Autodesk Inventor part; units mm, degrees
ref_plane "Work Plane1" through (-28.4804, 33.3109, -32.5631) normal (-1, 0, 0) x (0, 0, 1)
ref_plane "YZ Plane" through (0, 0, 0) normal (1, 0, 0) x (0, 1, 0)
ref_plane "XZ Plane" through (0, 0, 0) normal (0, 1, 0) x (-1, 0, 0)
sketch "Sketch1" plane through (0, 0, 0) normal (0, 0, 1) x (1, 0, 0)
  line L0 (6.9956, 3.6314) -> (6.4167, 3.8711)
  line L1 (5.7956, 3.9529) -> (6.4167, 3.8711)
  line L2 (5.1744, 3.8711) -> (5.7956, 3.9529)
  line L3 (4.5956, 3.6314) -> (5.1744, 3.8711)
  line L4 (4.0985, 3.25) -> (4.5956, 3.6314)
  line L5 (3.7171, 2.7529) -> (4.0985, 3.25)
  line L6 (3.4773, 2.1741) -> (3.7171, 2.7529)
  line L7 (3.4773, 2.1741) -> (3.3956, 1.5529)
  line L8 (3.4773, 0.9317) -> (3.3956, 1.5529)
  line L9 (3.4773, 0.9317) -> (3.7171, 0.3529)
  line L10 (3.7171, 0.3529) -> (4.0985, -0.1441)
  line L11 (4.0985, -0.1441) -> (4.5956, -0.5255)
  line L12 (4.5956, -0.5255) -> (5.1744, -0.7653)
  line L13 (5.1744, -0.7653) -> (5.7956, -0.8471)
  line L14 (5.7956, -0.8471) -> (6.4167, -0.7653)
  line L15 (6.4167, -0.7653) -> (6.9956, -0.5255)
  line L16 (6.9956, -0.5255) -> (7.4926, -0.1441)
  line L17 (7.4926, -0.1441) -> (7.874, 0.3529)
  line L18 (8.1138, 0.9317) -> (7.874, 0.3529)
  line L19 (8.1138, 0.9317) -> (8.1956, 1.5529)
  line L20 (8.1956, 1.5529) -> (8.1138, 2.1741)
  line L21 (8.1138, 2.1741) -> (7.874, 2.7529)
  line L22 (7.874, 2.7529) -> (7.4926, 3.25)
  line L23 (6.9956, 3.6314) -> (7.4926, 3.25)
  line L24 (6.7956, 1.5529) -> (6.7615, 1.8117)
  line L25 (6.7615, 1.2941) -> (6.7956, 1.5529)
  line L26 (6.6616, 1.0529) -> (6.7615, 1.2941)
  line L27 (6.5027, 0.8458) -> (6.6616, 1.0529)
  line L28 (6.2956, 0.6869) -> (6.5027, 0.8458)
  line L29 (6.0544, 0.587) -> (6.2956, 0.6869)
  line L30 (5.7956, 0.5529) -> (6.0544, 0.587)
  line L31 (5.5367, 0.587) -> (5.7956, 0.5529)
  line L32 (5.2956, 0.6869) -> (5.5367, 0.587)
  line L33 (5.0884, 0.8458) -> (5.2956, 0.6869)
  line L34 (4.9295, 1.0529) -> (5.0884, 0.8458)
  line L35 (4.8296, 1.2941) -> (4.9295, 1.0529)
  line L36 (4.7956, 1.5529) -> (4.8296, 1.2941)
  line L37 (4.7956, 1.5529) -> (4.8296, 1.8117)
  line L38 (4.8296, 1.8117) -> (4.9295, 2.0529)
  line L39 (4.9295, 2.0529) -> (5.0884, 2.26)
  line L40 (5.0884, 2.26) -> (5.2956, 2.4189)
  line L41 (5.2956, 2.4189) -> (5.5367, 2.5188)
  line L42 (5.5367, 2.5188) -> (5.7956, 2.5529)
  line L43 (5.7956, 2.5529) -> (6.0544, 2.5188)
  line L44 (6.0544, 2.5188) -> (6.2956, 2.4189)
  line L45 (6.2956, 2.4189) -> (6.5027, 2.26)
  line L46 (6.5027, 2.26) -> (6.6616, 2.0529)
  line L47 (6.6616, 2.0529) -> (6.7615, 1.8117)
  circle A0 centre (5.7956, 1.5529) radius 2.5
  arc A1 (1.7956, 7.8972) -> (9.7955, 7.8972) centre (5.7956, 1.5529) ccw
  line L48 (-28.4804, 55.5109) -> (-15.9804, 55.5109)
  line L49 (-28.4804, 55.5109) -> (-28.4804, 40.3109)
  line L50 (-15.9804, 40.3109) -> (-28.4804, 40.3109)
  line L51 (-15.9804, 40.3109) -> (-15.9804, 55.5109)
  line L52 (-20.6474, 51.7815) -> (-20.6304, 51.9109)
  line L53 (-20.6974, 51.6609) -> (-20.6474, 51.7815)
  line L54 (-20.7768, 51.5573) -> (-20.6974, 51.6609)
  line L55 (-20.8804, 51.4779) -> (-20.7768, 51.5573)
  line L56 (-21.001, 51.4279) -> (-20.8804, 51.4779)
  line L57 (-21.1304, 51.4109) -> (-21.001, 51.4279)
  line L58 (-21.2598, 51.4279) -> (-21.1304, 51.4109)
  line L59 (-21.3804, 51.4779) -> (-21.2598, 51.4279)
  line L60 (-21.4839, 51.5573) -> (-21.3804, 51.4779)
  line L61 (-21.5634, 51.6609) -> (-21.4839, 51.5573)
  line L62 (-21.5634, 51.6609) -> (-21.6133, 51.7815)
  line L63 (-21.6133, 51.7815) -> (-21.6304, 51.9109)
  line L64 (-21.6304, 51.9109) -> (-21.6133, 52.0403)
  line L65 (-21.5634, 52.1609) -> (-21.6133, 52.0403)
  line L66 (-21.4839, 52.2645) -> (-21.5634, 52.1609)
  line L67 (-21.3804, 52.3439) -> (-21.4839, 52.2645)
  line L68 (-21.3804, 52.3439) -> (-21.2598, 52.3939)
  line L69 (-21.2598, 52.3939) -> (-21.1304, 52.4109)
  line L70 (-21.1304, 52.4109) -> (-21.001, 52.3939)
  line L71 (-21.001, 52.3939) -> (-20.8804, 52.3439)
  line L72 (-20.8804, 52.3439) -> (-20.7768, 52.2645)
  line L73 (-20.7768, 52.2645) -> (-20.6974, 52.1609)
  line L74 (-20.6974, 52.1609) -> (-20.6474, 52.0403)
  line L75 (-20.6304, 51.9109) -> (-20.6474, 52.0403)
  line L76 (-21.7474, 51.7815) -> (-21.7304, 51.9109)
  line L77 (-21.7974, 51.6609) -> (-21.7474, 51.7815)
  line L78 (-21.8768, 51.5573) -> (-21.7974, 51.6609)
  line L79 (-21.9804, 51.4779) -> (-21.8768, 51.5573)
  line L80 (-22.101, 51.4279) -> (-21.9804, 51.4779)
  line L81 (-22.2304, 51.4109) -> (-22.101, 51.4279)
  line L82 (-22.3598, 51.4279) -> (-22.2304, 51.4109)
  line L83 (-22.4804, 51.4779) -> (-22.3598, 51.4279)
  line L84 (-22.5839, 51.5573) -> (-22.4804, 51.4779)
  line L85 (-22.6634, 51.6609) -> (-22.5839, 51.5573)
  line L86 (-22.6634, 51.6609) -> (-22.7133, 51.7815)
  line L87 (-22.7133, 51.7815) -> (-22.7304, 51.9109)
  line L88 (-22.7304, 51.9109) -> (-22.7133, 52.0403)
  line L89 (-22.6634, 52.1609) -> (-22.7133, 52.0403)
  line L90 (-22.5839, 52.2645) -> (-22.6634, 52.1609)
  line L91 (-22.4804, 52.3439) -> (-22.5839, 52.2645)
  line L92 (-22.4804, 52.3439) -> (-22.3598, 52.3939)
  line L93 (-22.3598, 52.3939) -> (-22.2304, 52.4109)
  line L94 (-22.2304, 52.4109) -> (-22.101, 52.3939)
  line L95 (-22.101, 52.3939) -> (-21.9804, 52.3439)
  line L96 (-21.9804, 52.3439) -> (-21.8768, 52.2645)
  line L97 (-21.8768, 52.2645) -> (-21.7974, 52.1609)
  line L98 (-21.7974, 52.1609) -> (-21.7474, 52.0403)
  line L99 (-21.7304, 51.9109) -> (-21.7474, 52.0403)
  line L100 (-22.8474, 51.7815) -> (-22.8304, 51.9109)
  line L101 (-22.8974, 51.6609) -> (-22.8474, 51.7815)
  line L102 (-22.9768, 51.5573) -> (-22.8974, 51.6609)
  line L103 (-23.0804, 51.4779) -> (-22.9768, 51.5573)
  line L104 (-23.201, 51.4279) -> (-23.0804, 51.4779)
  line L105 (-23.3304, 51.4109) -> (-23.201, 51.4279)
  line L106 (-23.4598, 51.4279) -> (-23.3304, 51.4109)
  line L107 (-23.5804, 51.4779) -> (-23.4598, 51.4279)
  line L108 (-23.6839, 51.5573) -> (-23.5804, 51.4779)
  line L109 (-23.7634, 51.6609) -> (-23.6839, 51.5573)
  line L110 (-23.7634, 51.6609) -> (-23.8133, 51.7815)
  line L111 (-23.8133, 51.7815) -> (-23.8304, 51.9109)
  line L112 (-23.8304, 51.9109) -> (-23.8133, 52.0403)
  line L113 (-23.7634, 52.1609) -> (-23.8133, 52.0403)
  line L114 (-23.6839, 52.2645) -> (-23.7634, 52.1609)
  line L115 (-23.5804, 52.3439) -> (-23.6839, 52.2645)
  line L116 (-23.5804, 52.3439) -> (-23.4598, 52.3939)
  line L117 (-23.4598, 52.3939) -> (-23.3304, 52.4109)
  line L118 (-23.3304, 52.4109) -> (-23.201, 52.3939)
  line L119 (-23.201, 52.3939) -> (-23.0804, 52.3439)
  line L120 (-23.0804, 52.3439) -> (-22.9768, 52.2645)
  line L121 (-22.9768, 52.2645) -> (-22.8974, 52.1609)
  line L122 (-22.8974, 52.1609) -> (-22.8474, 52.0403)
  line L123 (-22.8304, 51.9109) -> (-22.8474, 52.0403)
  line L124 (-21.6304, 37.8109) -> (-21.6304, 40.3109)
  line L125 (-15.9804, 37.8109) -> (-21.6304, 37.8109)
  line L126 (-15.9804, 37.8109) -> (-15.9804, 40.3109)
  line L127 (-21.6304, 40.3109) -> (-15.9804, 40.3109)
  line L128 (-28.4804, 37.8109) -> (-28.4804, 40.3109)
  line L129 (-22.8304, 37.8109) -> (-28.4804, 37.8109)
  line L130 (-22.8304, 37.8109) -> (-22.8304, 40.3109)
  line L131 (-28.4804, 40.3109) -> (-22.8304, 40.3109)
  line L132 (-28.4804, 40.3109) -> (-15.9804, 40.3109)
  line L133 (-15.9804, 40.3109) -> (-15.9804, 45.3109)
  line L134 (-15.9804, 45.3109) -> (-28.4804, 45.3109)
  line L135 (-28.4804, 45.3109) -> (-28.4804, 40.3109)
  line L136 (-15.9804, 45.3109) -> (-12.9804, 45.3109)
  line L137 (-12.9804, 45.3109) -> (-12.9804, 40.3109)
  line L138 (-12.9804, 40.3109) -> (-15.9804, 40.3109)
  line L139 (-15.9804, 40.3109) -> (-15.9804, 45.3109)
  line L140 (-28.4804, 45.3109) -> (-31.4804, 45.3109)
  line L141 (-31.4804, 45.3109) -> (-31.4804, 40.3109)
  line L142 (-31.4804, 40.3109) -> (-28.4804, 40.3109)
  line L143 (-28.4804, 40.3109) -> (-28.4804, 45.3109)
  line L144 (-12.9804, 45.3109) -> (5.7956, 45.3109)
  line L145 (1.7956, 40.3109) -> (-12.9804, 40.3109)
  line L146 (-12.9804, 40.3109) -> (-12.9804, 45.3109)
  line L147 (9.7956, 45.3109) -> (9.7955, 7.8972)
  line L148 (1.7956, 7.8972) -> (1.7956, 40.3109)
  line L149 (1.7956, 45.3109) -> (9.7956, 45.3109)
  line L150 (9.7956, 45.3109) -> (1.7956, 3.9529) construction
  line L151 (9.7956, 3.9529) -> (1.7956, 45.3109) construction
  line L152 (5.7956, 4.0529) -> (5.7956, 3.9529)
  line L153 (5.7956, 1.5529) -> (-36.8703, 1.5529)
  line L154 (-22.2304, 45.3109) -> (-22.2304, 1.5529)
  line L155 (1.7956, 39.0609) -> (1.7956, 45.3109)
  point P0 (0, 0)
  point P1 (5.7956, 24.6319)
  dimension "d0" = 5
  dimension "d1" = 15
  dimension "d2" = 5
  dimension "d3" = 3
  dimension "d4" = 3
  dimension "d6" = 8
extrude "Extrusion1" add sketch "Sketch1" along normal blind 3 contours A1 L148 L155 L144 L149 L147
sketch "Sketch2" plane through (1.7956, 39.0609, 0) normal (-1, 0, 0) x (0, 0, 1)
  line L0 (-5.2631, 16.45) -> (-5.2631, 1.25)
  line L1 (-27.7631, 1.25) -> (-27.7631, 16.45)
  line L2 (-5.2631, 16.45) -> (-27.7631, 16.45)
  line L3 (-27.7631, 1.25) -> (-27.7631, 16.45)
  line L4 (-27.7631, 1.25) -> (-32.5631, 1.25)
  line L5 (-32.5631, 1.25) -> (-32.5631, -1.25)
  line L6 (-27.7631, -1.25) -> (-32.5631, -1.25)
  line L7 (-27.7631, -1.25) -> (-27.7631, -5.75)
  line L8 (-5.2631, -5.75) -> (-27.7631, -5.75)
  line L9 (-5.2631, -1.25) -> (-5.2631, -5.75)
  line L10 (-5.2631, -1.25) -> (-0.4631, -1.25)
  line L11 (-0.4631, -1.25) -> (-0.4631, 1.25)
  line L12 (-5.2631, 1.25) -> (-0.4631, 1.25)
  line L13 (-5.2631, 16.45) -> (-5.2631, 1.25)
  line L14 (0, 6.25) -> (0, 0)
  line L15 (-27.7631, 1.25) -> (0, 1.25)
  line L16 (0, 1.25) -> (0, 6.25)
  line L17 (0, 6.25) -> (-27.7631, 6.25)
  line L18 (-27.7631, 6.25) -> (-27.7631, 1.25)
  line L19 (-27.7631, 6.25) -> (-30.7631, 6.25)
  line L20 (-30.7631, 6.25) -> (-30.7631, 1.25)
  line L21 (-30.7631, 1.25) -> (-27.7631, 1.25)
  line L22 (-27.7631, 1.25) -> (-27.7631, 6.25)
  point P0 (0, -39.0609)
  dimension "d9" = 3
ref_plane "Work Plane1" through (-28.4804, 33.3109, -32.5631) normal (-1, 0, 0) x (0, 0, 1)
extrude "Extrusion2" add sketch "Sketch2" against normal blind 15.5 from surface at 30.276 contours L17 L14 L15 L12 L0 | L0 L15 L1 L17
sketch "Sketch3" plane through (-12.9804, 40.3109, 0) normal (1, 0, 0) x (0, 0, -1)
  line L0 (0, -32.4137) -> (0, 5)
  line L1 (0, 5) -> (-3, 5)
  line L2 (-3, -32.4137) -> (-3, 5)
  line L3 (0, -32.4137) -> (-3, -32.4137)
  line L4 (0, 5) -> (0, 0)
  line L5 (0, 0) -> (27.7631, 0)
  line L6 (27.7631, 0) -> (27.7631, 5)
  line L7 (27.7631, 5) -> (0, 5)
  line L8 (27.7631, 5) -> (0, 5)
  line L9 (0, 0) -> (3, 0)
  line L10 (3, 0) -> (3, 5)
  line L11 (3, 5) -> (0, 5)
  line L12 (0, 5) -> (0, 0)
  point P0 (0, -40.3109)
  dimension "d12" = 3
extrude "Extrusion3" add sketch "Sketch3" along normal up to surface (22.776 mm away) contours L0 L7 L10 L5
properties part number "armV"
Here's how the part is built. I have some questions about the finished solid (model axes, mm). A direction names the side the tool comes from. Round coordinates to 2 decimals unless told otherwise and drop trailing zeros. Write each loop counter-clockwise with the first axis right and the second up, starting at its lowest first coordinate (ties: lowest second). Pieces come first, ordered by that corner, then holes.
1. I need wall thicknesses on L1, parallel to Z at x = -1.5, y = 1; L2, parallel to X at y = 22, z = 1.5; L3, parallel to Z at x = -15.5, y = 42. Which ranges of each line are inside material? Lowest first, please.
2. Suppose I cut it at C-C (x = -7). List the corners of the cut face in (y, z) for me, and give its area (3 significant figures).
3. Suppose I cut it at B-B (x = 1). List the corners of the cut face in (y, z) for me, and give its area (3 significant figures).
4. Suppose I cut it at D-D (z = -17.5). List the corners of the cut face in (x, y) for me.
5. If we mould it in two halves opening along X, with no side actions, what happens to faces 4 (the flat face through (-18, 45.311, -13)), 5 (the cylindrical face through (6.066, -5.942, 1.479)), 6 (the flat face through (1.796, 26, 1)), 7 (the cylindrical face through (8.18, 0.8, 1.48))? For each: released by +X, released by -X, zero draft, split by the parting line, or undercut.
6. Suppose I cut it at A-A (y = 3). List the corners of the cut face in (x, z) for me.
7. Will these pins go through, and if not, where does the flat tip stop? pin 1 Ø0.9 at (y, z) = (36, 1.5) entering from -X; pin 2 Ø7.5 at (x, y) = (5, 14.5) entering from -Z; pin 3 Ø5.5 at (x, y) = (-1, 43) entering from -Z.
8. For faces 1 (the flat face through (-2, 43, -3)), 2 (the flat face through (-21, 43, -27.763)), 3 (the flat face through (6, 18, 0)), which set-ups out of +Z, -Z, +X, -X, +Y, -Y let a thin tool reach every point of the face, with its end or its side?
Answer sheet:
1. L1: z = 0 to 3
1. L2: x = 1.8 to 9.8
1. L3: z = -27.76 to 0
2. outline: (40.31, -3) - (45.31, -3) - (45.31, 0) - (40.31, 0) - close
2. area: 15.0 mm2
3. outline: (-4.21, 0) - (7.32, 0) - (7.32, 3) - (-4.21, 3) - close; (40.31, -3) - (45.31, -3) - (45.31, 0) - (40.31, 0) - close
3. area: 49.6 mm2
4. outline: (-28.48, 40.31) - (-12.98, 40.31) - (-12.98, 45.31) - (-28.48, 45.31) - close
5. face 4: zero draft
5. face 5: split by the parting line
5. face 6: released by -X
5. face 7: undercut
6. outline: (-1.56, 0) - (3.76, 0) - (3.76, 3) - (-1.56, 3) - close; (7.83, 0) - (13.15, 0) - (13.15, 3) - (7.83, 3) - close
7. pin 1: stops at x = 1.8
7. pin 2: stops at z = 0
7. pin 3: stops at z = -3
8. face 1: -Z, +X, +Y, -Y
8. face 2: -Z, +X, -X, +Y, -Y
8. face 3: -Z, +X, -X, -Y
